Design review of the part built by this model. Coordinates are the model's own, in mm. A direction names the side the tool comes from. Coordinates: 2 decimals unless noted, no trailing zeros. Loops run counter-clockwise (first coordinate to the right, second up) from the corner with the lowest first, then second, coordinate; pieces in that order, holes last. Notation, with made-up numbers: (1.5, -26.5) - (8.5, -26.5) arc R24 ccw to (8.5, 10.5) - close; hole circle Ø8 at (10, 5). An arc over 180 degrees is marked (long way). One line per question, with ' | ' between items.
from build123d import *

# Parameters (mm, degrees)
SKETCH1_R           = 12.7
BOSS_EXTRUDE1_DEPTH = 7.9248
SKETCH2_R           = 9.525
BOSS_EXTRUDE2_DEPTH = 1.524
BOSS_EXTRUDE4_START = 6.35
SKETCH4_R           = 9.525
BOSS_EXTRUDE4_DEPTH = 6.35
SKETCH5_R           = 8.636
BOSS_EXTRUDE5_DEPTH = 9.525
SKETCH6_R           = 6.35
CUT_EXTRUDE1_DEPTH  = 25.4


with BuildPart() as part:
    # Sketch1 → Boss-Extrude1 (new body)
    with BuildSketch(Plane(origin=(0, 0, 0), x_dir=(0, 0, -1), z_dir=(1, 0, 0))):
        Circle(SKETCH1_R)
    extrude(amount=BOSS_EXTRUDE1_DEPTH)

    # Sketch2 → Boss-Extrude2 (add)
    with BuildSketch(Plane(origin=(7.9248, 0, 0), x_dir=(0, 0, -1), z_dir=(1, 0, 0))):
        with Locations(Location((0, 0, 0), (0, 0, 180))):
            Circle(SKETCH2_R)
    extrude(amount=BOSS_EXTRUDE2_DEPTH)

    # Sketch4 → Boss-Extrude4 (add)
    with BuildSketch(Plane.ZY.offset(BOSS_EXTRUDE4_START)):
        Circle(SKETCH4_R)
    extrude(amount=-BOSS_EXTRUDE4_DEPTH)

    # Sketch5 → Boss-Extrude5 (add)
    with BuildSketch(Plane.ZY.offset(6.35)):
        with Locations(Location((0, 0, 0), (0, 0, 180))):
            Circle(SKETCH5_R)
    extrude(amount=BOSS_EXTRUDE5_DEPTH)

    # Sketch6 → Cut-Extrude1 (cut)
    with BuildSketch(Plane.ZY.offset(15.875)):
        Circle(SKETCH6_R)
    extrude(amount=-CUT_EXTRUDE1_DEPTH, mode=Mode.SUBTRACT)


solid = part.part
Q1. Draft analysis for pull direction Y (two halves, no side actions). For faces 4 (the cylindrical face through (-3.219, -5.796, -7.559)), 5 (the flat face through (-15.875, -5, 5)), 6 (the cylindrical face through (-3.39, -6.2, -1.38)), state which applies: +Y half, -Y half, draft (parallel to the pull), parting line (faces both ways), or undercut.
Returned:
face 4: parting line | face 5: draft | face 6: undercut
Q2. Take a section at A-A (z = 0). Give the boundary of the cut face in (x, y) (3 decimals).
Returned:
outline: (-15.875, -8.636) - (-6.35, -8.636) - (-6.35, -9.525) - (0, -9.525) - (0, -12.7) - (7.925, -12.7) - (7.925, -9.525) - (9.449, -9.525) - (9.449, -6.35) - (-15.875, -6.35) - close; (-15.875, 6.35) - (9.449, 6.35) - (9.449, 9.525) - (7.925, 9.525) - (7.925, 12.7) - (0, 12.7) - (0, 9.525) - (-6.35, 9.525) - (-6.35, 8.636) - (-15.875, 8.636) - close
Q3. Take a section at D-D (y = 8). Give the boundary of the cut face in (x, z) (3 decimals), plus the area to 3 significant figures.
Returned:
outline: (-15.875, -3.253) - (-6.35, -3.253) - (-6.35, -5.17) - (0, -5.17) - (0, -9.864) - (7.925, -9.864) - (7.925, -5.17) - (9.449, -5.17) - (9.449, 5.17) - (7.925, 5.17) - (7.925, 9.864) - (0, 9.864) - (0, 5.17) - (-6.35, 5.17) - (-6.35, 3.253) - (-15.875, 3.253) - close | area: 300 mm²
Q4. To check wall thickness, follow line 1 along Y through (x, z) = (-7.25, 0); line 2 along Y through (x, z) = (-2, 0) (3 decimals); line 3 along X through (y, z) = (8.25, -9.25). State the ranges of each line that lie inside material, in increasing order.
Returned:
line 1: y = -8.64 to -6.35, 6.35 to 8.64 | line 2: y = -9.525 to -6.35, 6.35 to 9.525 | line 3: x = 0 to 7.92
Q5. For pin 1 (3 mm diameter, centred on x = 6.5, y = 9.5, fed in from +Z); pin 2 (2 mm diameter, centred on y = 10, z = 5.5, fed in from -X); pin 3 (3 mm diameter, centred on x = -7, y = -7, fed in from +Z), all flat-tipped, find the tip position at first contact; note any pin that passes through.
Returned:
pin 1: stops at z = 9.86 | pin 2: stops at x = 0 | pin 3: stops at z = 7.67
Q6. Take a section at C-C (x = 2.25). Give the boundary of the cut face in (y, z), plus the area to 3 significant figures.
Returned:
outline: circle Ø25.4 at (0, 0); hole circle Ø12.7 at (0, 0) | area: 380 mm²
Q7. Tool access review of faces 1 (the flat face through (7.925, 9, -5)), 2 (the cylindrical face through (-11.046, -8.563, 1.124)), 3 (the flat face through (9.449, 6.2, 2)): name each direction out of +Z, -Z, +X, -X, +Y, -Y from which nothing blocks a thin tool from reaching the whole face with its end or side.
Returned:
face 1: +X | face 2: -X | face 3: +Z, -Z, +X, +Y, -Y
